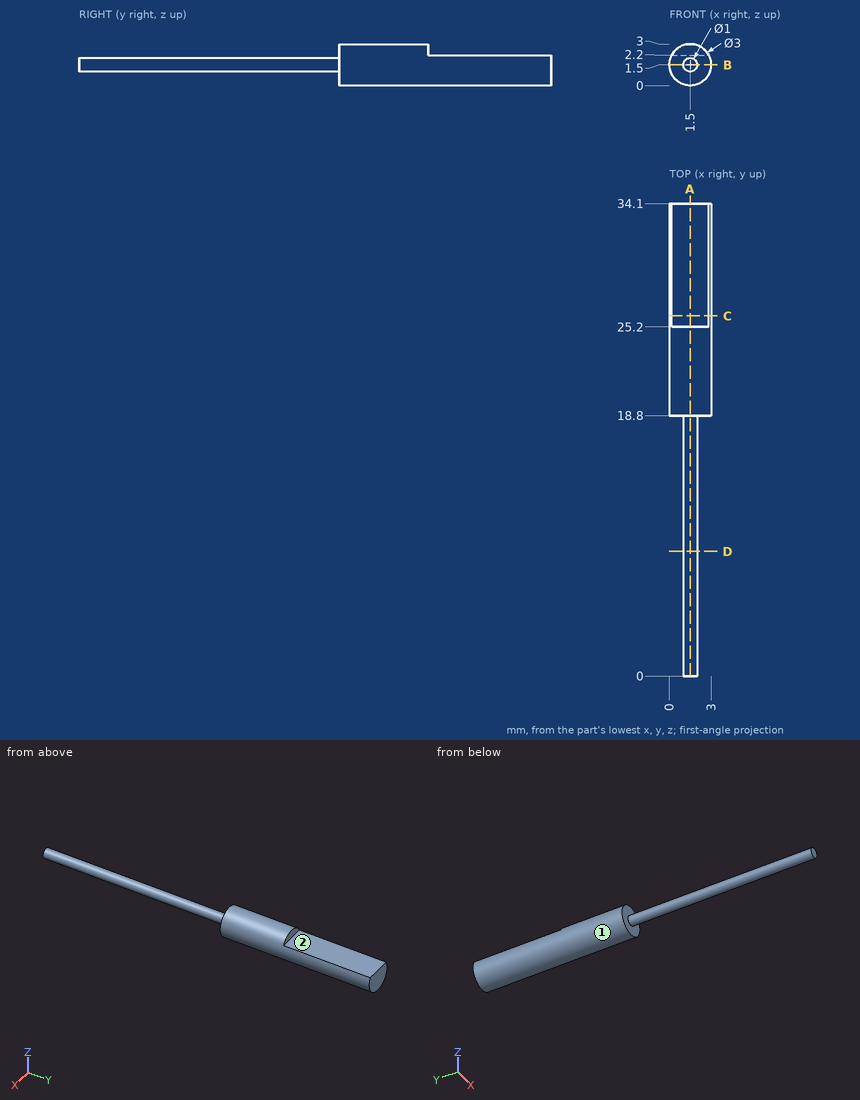
Verification items for this drawing (mm, ordinates from the low corner). A direction names the side the tool comes from. Round coordinates to 2 decimals unless told otherwise and drop trailing zeros. Order: outer loops, then holes, each group sorted by start corner. A loop starts at its lowest first (then second) coordinate and runs counter-clockwise, first axis right, second up. Notation, with made-up numbers: (-8.5, -26) - (49.5, -26) arc R28 cw to (49.5, 0) - close; hole circle Ø11 at (77.5, 26.25). An arc over 180 degrees is marked (long way). Use CSV: the item, a comma, the result in double quotes. Start each with the question number.
1) Section check C-C, the plane y = 26. Record the cut outline in (x, z).
2) Go/stop test with flat-tipped pins: P1, Ø1.5, axis at y = 10, z = 1, coming from the -X side; P2, Ø1.3, axis at x = 2, y = 29, coming from the +Z side. Record where each tip stops, or that it passes through.
3) Section check D-D, the plane y = 9. Record the cut outline in (x, z), plus the area to 3 significant figures.
4) Section check B-B, the plane z = 1.5. Record the cut outline in (x, y), plus the area to 3 significant figures.
5) Thickness scan on L1, parallel to X at y = 30, z = 0.8; L2, parallel to Y at x = 0.3, z = 1.15. Record the ranges inside material, lowest first.
6) Access from +Z, -Z, +X, -X, +Y, -Y to the whole of each face (thin tool, end or side, straight path). Record for the marked faces 1 and 2.
7) Section check A-A, the plane x = 1.5. Record the cut outline in (y, z).
Answers:
1,outline,"(0.17, 2.2) arc R1.5 ccw (long way) to (2.83, 2.2) - close"
2,P1,"stops at x = 1"
2,P2,"stops at z = 2.2"
3,outline,"circle Ø1 at (1.5, 1.5)"
3,area,"0.785 mm²"
4,outline,"(0, 18.8) - (1, 18.8) - (1, 0) - (2, 0) - (2, 18.8) - (3, 18.8) - (3, 34.1) - (0, 34.1) - close"
4,area,"64.7 mm²"
5,L1,"x = 0.17 to 2.83"
5,L2,"y = 18.8 to 34.1"
6,face 1,"+Y, -Y"
6,face 2,"+Z, +X, -X, +Y"
7,outline,"(0, 1) - (18.8, 1) - (18.8, 0) - (34.1, 0) - (34.1, 2.2) - (25.2, 2.2) - (25.2, 3) - (18.8, 3) - (18.8, 2) - (0, 2) - close"
